The figure shows three views and two pictorial views of one solid part (mm, origin at its lowest corner). Answer the questions. A direction names the side the tool comes from. Coordinates: 2 decimals unless noted, no trailing zeros. Loops run counter-clockwise (first coordinate to the right, second up) from the corner with the lowest first, then second, coordinate; pieces in that order, holes last. Notation, with made-up numbers: (40, 19) - (83, 19) arc R16 cw to (83, 36) - close; hole circle Ø7 at (55, 59). An arc over 180 degrees is marked (long way). One line per question, with ' | ' between items.
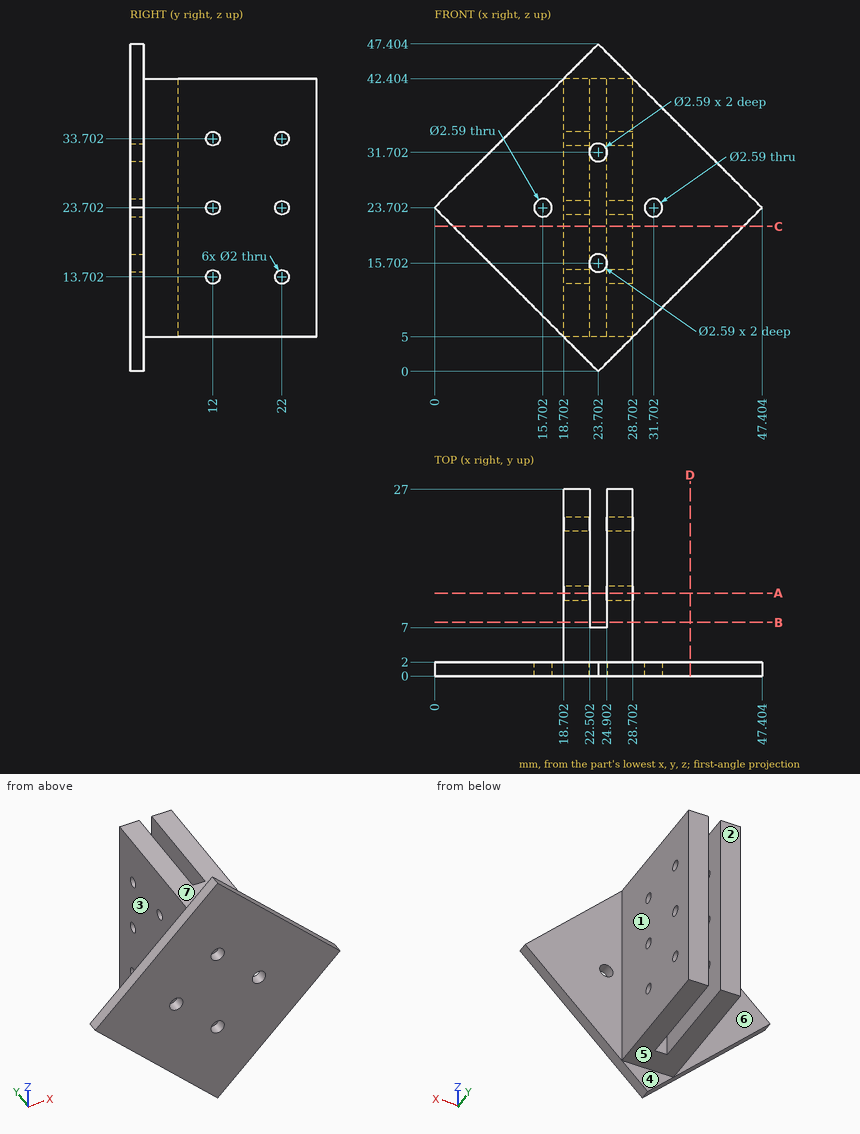
Item 1: Each of these flat-tipped pins is pushed along its axis until it touches: pin 1 Ø10 at (y, z) = (19.5, 32.5) entering from -X; pin 2 Ø1.5 at (x, y) = (19.5, 11) entering from -Z; pin 3 Ø3 at (y, z) = (22, 33.7) entering from +X; pin 4 Ø1.2 at (y, z) = (12, 23.7) entering from +X. Where does it stop, or does it pass through?
Taken from the geometry:
pin 1: stops at x = 18.7 | pin 2: stops at z = 5 | pin 3: stops at x = 28.7 | pin 4: passes through
Item 2: Find section A-A, the plane y = 12. State how many separate pieces and enclosed holes the cut face has, plus the area to 3 significant figures.
Taken from the geometry:
separate pieces: 8 | enclosed holes: 0 | area: 239 mm2
Item 3: Find section D-D, the plane x = 37. Write down the section's boundary in (y, z) (1 decimal).
Taken from the geometry:
outline: (0, 13.3) - (2, 13.3) - (2, 34.1) - (0, 34.1) - close
Item 4: The mould has two halves that part along Z. Classify the marked faces 5, 6 and 7: pulls with the +Z half, pulls with the -Z half, needs draft (parallel to the pull), parting line crosses it, or undercut.
Taken from the geometry:
face 5: pulls with the -Z half | face 6: needs draft | face 7: pulls with the +Z half
Item 5: Find section C-C, the plane z = 21. Write down the section's boundary in (x, y), plus the area to 3 significant figures.
Taken from the geometry:
outline: (2.7, 0) - (44.7, 0) - (44.7, 2) - (28.7, 2) - (28.7, 27) - (24.9, 27) - (24.9, 7) - (22.5, 7) - (22.5, 27) - (18.7, 27) - (18.7, 2) - (2.7, 2) - close | area: 286 mm2
Item 6: Find the intervals of material crossed by line 1 (Z direction, x = 26.35, y = 12); line 2 (X direction, y = 20.5, z = 19); line 3 (X direction, y = 4.75, z = 24), in increasing order. Write a range as [from, to].
Taken from the geometry:
line 1: z = [5, 12.7], [14.7, 22.7], [24.7, 32.7], [34.7, 42.4] | line 2: x = [18.7, 22.5], [24.9, 28.7] | line 3: x = [18.7, 28.7]
Item 7: Which of the six approach directions +Z, -Z, +X, -X, +Y, -Y give full straight-line access (tool end or side, diameter ignored) to the marked faces 1, 2, 3 and 4?
Taken from the geometry:
face 1: +Z, -Z, +X, +Y | face 2: +Z, -Z, +X, -X, +Y | face 3: +Z, -Z, -X, +Y | face 4: -Z, +X, -X, +Y
Item 8: Find section B-B, the plane y = 7.75. Write down the section's boundary in (x, z), plus the area to 3 significant figures.
Taken from the geometry:
outline: (18.7, 5) - (22.5, 5) - (22.5, 42.4) - (18.7, 42.4) - close; (24.9, 5) - (28.7, 5) - (28.7, 42.4) - (24.9, 42.4) - close | area: 284 mm2
